For this review, take the finished solid that the model builds, in its own axes (mm). Coordinates: 2 decimals unless noted, no trailing zeros. Order: outer loops, then holes, each group sorted by start corner. A loop starts at its lowest first (then second) coordinate and runs counter-clockwise, first axis right, second up.
from build123d import *

# Parameters (mm, degrees)
TOP_FIREWALL_DEPTH = 1


# Sheet-metal steps are written as plain solids
with BuildPart() as part:
    # Sketch1 → Top Firewall (new body)
    with BuildSketch(Plane.XY):
        with BuildLine():
            Line((-370, 37.570353211), (-370, 0))
            Line((-370, 0), (370, 0))
            Line((370, 0), (370, 37.570353211))
            ThreePointArc((370, 37.570353211), (368.537307916, 56.249395802), (364.184889464, 74.473076931))
            Line((364.184889464, 74.473076931), (287.42, 312))
            Line((287.42, 312), (-287.42, 312))
            Line((-287.42, 312), (-364.184889464, 74.473076931))
            ThreePointArc((-364.184889464, 74.473076931), (-368.537307916, 56.249395802), (-370, 37.570353211))
        make_face()
    extrude(amount=-TOP_FIREWALL_DEPTH)


solid = part.part
1. To check wall thickness, follow L1, parallel to X at y = 42.5, z = -0.3; L2, parallel to X at y = 240, z = -0.2. State the ranges of each line that lie inside material, in increasing order.
Answer below:
L1: x = -369.9 to 369.9
L2: x = -310.69 to 310.69
2. Take a section at B-B, the plane x = 324. Give the boundary of the cut face in (y, z).
Answer below:
outline: (0, -1) - (198.81, -1) - (198.81, 0) - (0, 0) - close
3. Take a section at A-A, the plane z = -0.6. Give the boundary of the cut face in (x, y), plus the area to 3 significant figures.
Answer below:
outline: (-370, 0) - (370, 0) - (370, 37.57) arc R120 ccw to (364.18, 74.47) - (287.42, 312) - (-287.42, 312) - (-364.18, 74.47) arc R120 ccw to (-370, 37.57) - close
area: 210,000 mm2
4. The part is to be moulded in two halves that separate along Y. For faces 1 (the face through (326.34, 191.57, -0.49)), 2 (the face through (-5, 158, -1)), say which applies: +Y half, -Y half, draft (parallel to the pull), parting line (faces both ways), or undercut.
Answer below:
face 1: +Y half
face 2: draft
5. Take a section at C-C, the plane y = 82. Give the boundary of the cut face in (x, z).
Answer below:
outline: (-361.75, -1) - (361.75, -1) - (361.75, 0) - (-361.75, 0) - close
